Here's the drawing with two shaded views (mm, measured from the low corner). I have some questions. Round coordinates to 2 decimals unless told otherwise and drop trailing zeros. Order: outer loops, then holes, each group sorted by start corner. A loop starts at its lowest first (then second) coordinate and runs counter-clockwise, first axis right, second up.
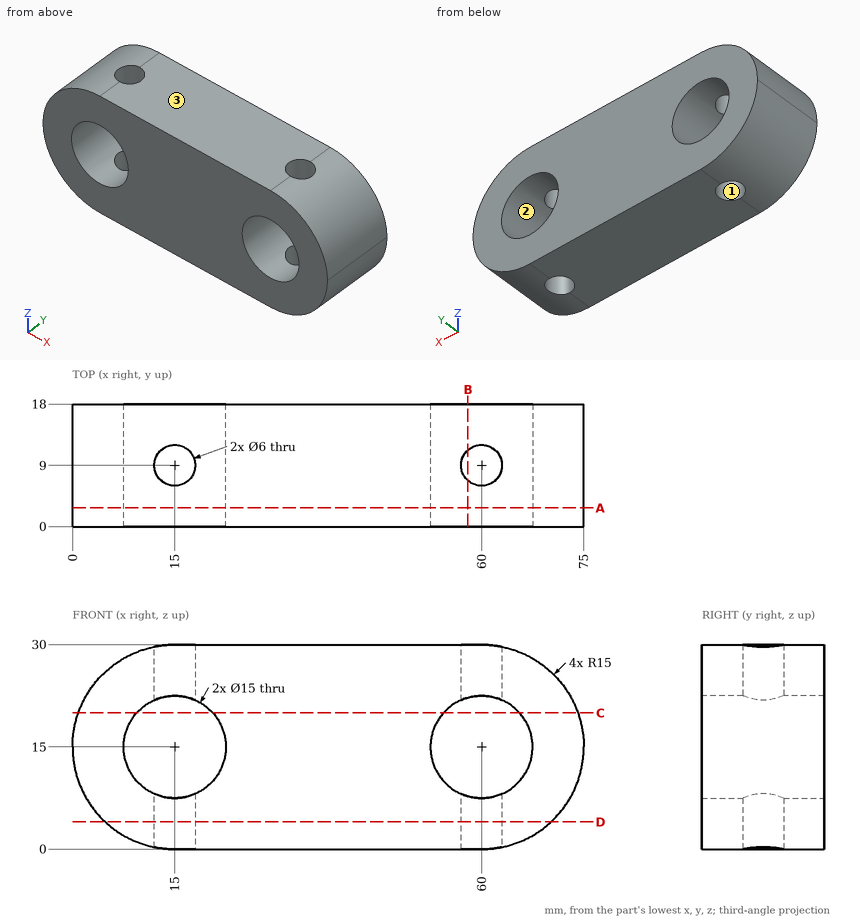
1. If we mould it in two halves opening along Z, with no side actions, what happens to the marked faces 1, 2 and 3? For each: released by +Z, released by -Z, zero draft, split by the parting line, or undercut.
Evaluation:
face 1: zero draft
face 2: undercut
face 3: released by +Z
2. If we section it at D-D, the plane z = 4: Write out the boundary of the cut face in (x, y).
Evaluation:
outline: (4.8, 0) - (70.2, 0) - (70.2, 18) - (4.8, 18) - close; hole circle Ø6 at (15, 9); hole circle Ø6 at (60, 9)
3. If we section it at A-A, the plane y = 2.75: State how many separate pieces and enclosed holes the cut face has, and give its area (3 significant figures).
Evaluation:
separate pieces: 1
enclosed holes: 2
area: 1,700 mm2
4. If we section it at C-C, the plane z = 20: Write out the boundary of the cut face in (x, y), and give its area (3 significant figures).
Evaluation:
outline: (0.86, 0) - (9.41, 0) - (9.41, 18) - (0.86, 18) - close; (20.59, 0) - (54.41, 0) - (54.41, 18) - (20.59, 18) - close; (65.59, 0) - (74.14, 0) - (74.14, 18) - (65.59, 18) - close
area: 917 mm2
5. I'm going to push flat-ended pins straight in: P1, Ø4, axis at y = 13.5, z = 11.5, coming from the +X side; P2, Ø6, axis at y = 13.5, z = 10, coming from the -X side; P3, Ø8, axis at y = 2.5, z = 19.5, coming from the -X side. Where does each tip first touch, or does it pass through?
Evaluation:
P1: stops at x = 74.92
P2: stops at x = 0.13
P3: stops at x = 0.01
6. If we section it at B-B, the plane x = 58: Write out the boundary of the cut face in (y, z).
Evaluation:
outline: (0, 0) - (6.76, 0) - (6.76, 7.77) - (0, 7.77) - close; (0, 22.23) - (6.76, 22.23) - (6.76, 30) - (0, 30) - close; (11.24, 0) - (18, 0) - (18, 7.77) - (11.24, 7.77) - close; (11.24, 22.23) - (18, 22.23) - (18, 30) - (11.24, 30) - close
7. I need wall thicknesses on probe 1 along X at (y, z) = (11.5, 15); probe 2 along X at (y, z) = (5.75, 11); probe 3 along Y at (x, z) = (15, 4.25). Which ranges of each line are inside material? Lowest first, please.
Evaluation:
probe 1: x = 0 to 7.5, 22.5 to 52.5, 67.5 to 75
probe 2: x = 0.54 to 8.66, 21.34 to 53.66, 66.34 to 74.46
probe 3: y = 0 to 6, 12 to 18
